Read the model definition and answer for the solid it produces. Units are mm, in the model's axes. A direction names the side the tool comes from. Coordinates: 2 decimals unless noted, no trailing zeros.
1) Each of these flat-tipped pins is pushed along its axis until it touches: pin 1 Ø15 at (x, y) = (-283.5, 99) entering from -Z; pin 2 Ø25 at (y, z) = (9.5, -34.5) entering from +X; pin 3 Ø15 at (y, z) = (-68.5, -71) entering from +X. Where does it stop, or does it pass through?
2) Find the intervals of material crossed by line 1 (Y direction, x = 168, z = -93); line 2 (Z direction, x = 123, y = 245), in increasing order.
3) The part is cut by section A-A (x = -170). Give the number of separate pieces and of enclosed holes in the cut face, then the cut area to 3 significant figures.
4) Determine the mould class of faces 1 (the face through (-300, -4, -25)), 2 (the face through (-4, 300, -25)), 3 (the face through (-5.91, 263.52, -677.54)), 4 (the face through (260.71, -239.53, -421.67)) for opening direction Y: +Y half, -Y half, draft (parallel to the pull), parting line (faces both ways), or undercut.
5) Which of the six approach directions +Z, -Z, +X, -X, +Y, -Y give full straight-line access (tool end or side, diameter ignored) to faces 5 (the face through (-254.688, -3, -75)), 6 (the face through (300, -4, -25)), 7 (the face through (3.72, -263.415, -676.431)), 8 (the face through (-295.762, 270.424, -751.192))?
from build123d import *

# Parameters (mm, degrees)
F0_W      = 50
F0_H      = 50
F2_W      = 50
F2_H      = 50
F3_W      = 600
F3_H      = 600
F8_DEPTH  = 50
F9_W      = 409.375
F9_H      = 409.375
F10_DEPTH = 50


with BuildPart() as f4:
    # F0 (on Top) → F4 section 0
    with BuildSketch(Plane.XY):
        with Locations((-225, -225)):
            Rectangle(F0_W, F0_H)
    # F2 (on offset) → F4 section 1
    with BuildSketch(Plane.XY.offset(-800)):
        with Locations((-300, -300)):
            Rectangle(F2_W, F2_H)
    loft()



with BuildPart() as f5:
    # F0 (on Top) → F5 section 0
    with BuildSketch(Plane.XY):
        with Locations((225, -225)):
            Rectangle(F0_W, F0_H)
    # F2 (on offset) → F5 section 1
    with BuildSketch(Plane.XY.offset(-800)):
        with Locations((300, -300)):
            Rectangle(F2_W, F2_H)
    loft()


with BuildPart() as f6:
    # F0 (on Top) → F6 section 0
    with BuildSketch(Plane.XY):
        with Locations((-225, 225)):
            Rectangle(F0_W, F0_H)
    # F2 (on offset) → F6 section 1
    with BuildSketch(Plane.XY.offset(-800)):
        with Locations((-300, 300)):
            Rectangle(F2_W, F2_H)
    loft()


with BuildPart() as f7:
    # F0 (on Top) → F7 section 0
    with BuildSketch(Plane.XY):
        with Locations((225, 225)):
            Rectangle(F0_W, F0_H)
    # F2 (on offset) → F7 section 1
    with BuildSketch(Plane.XY.offset(-800)):
        with Locations((300, 300)):
            Rectangle(F2_W, F2_H)
    loft()


with BuildPart() as f4_1:
    add(f4.part)

    add(f5.part)  # F8 merges F5

    add(f6.part)  # F8 merges F6

    add(f7.part)  # F8 merges F7
    # F3 (on Top) → F8 (join)
    with BuildSketch(Plane.XY):
        Rectangle(F3_W, F3_H)
    extrude(amount=-F8_DEPTH)

    # F9 (on face) → F10 (join)
    with BuildSketch(Plane(origin=(0, 0, -50), x_dir=(1, 0, 0), z_dir=(0, 0, -1))):
        Polygon((254.6875, -254.6875), (254.6875, -204.6875), (254.6875, 204.6875), (254.6875, 254.6875), (204.6875, 254.6875), (-204.6875, 254.6875), (-254.6875, 254.6875), (-254.6875, -254.6875), (-204.6875, -254.6875), (204.6875, -254.6875), align=None)
        Rectangle(F9_W, F9_H, mode=Mode.SUBTRACT)
    extrude(amount=F10_DEPTH)

    # F13 (on face) → F15 section 0
    with BuildSketch(Plane(origin=(-198.2575024201, 0, 18.5866408519), x_dir=(0, 1, 0), z_dir=(0.9956342261, 0, -0.0933407087))):
        Polygon((261.0594902568, -672.8252733026), (265.7063268379, -722.6088741144), (315.2744650336, -717.9821489666), (310.6276284526, -668.1985481548), align=None)
    # F14 (on face) → F15 section 1
    with BuildSketch(Plane(origin=(198.2575024201, 0, 18.5866408519), x_dir=(0, -1, 0), z_dir=(-0.9956342261, 0, -0.0933407087))):
        Polygon((-315.2744650336, -717.9821489666), (-265.7063268379, -722.6088741144), (-261.0594902568, -672.8252733026), (-310.6276284526, -668.1985481548), align=None)
    loft()

    # F12 (on face) → F18 section 0
    with BuildSketch(Plane(origin=(0, 198.2575024201, 18.5866408519), x_dir=(1, 0, 0), z_dir=(0, -0.9956342261, -0.0933407087))):
        Polygon((-315.7063268379, -722.6088741144), (-265.7063268379, -722.6088741144), (-261.0594902568, -672.8252733026), (-311.0594902568, -672.8252733026), align=None)
    # F16 (on face) → F18 section 1
    with BuildSketch(Plane(origin=(0, -198.2575024201, 18.5866408519), x_dir=(-1, 0, 0), z_dir=(0, 0.9956342261, -0.0933407087))):
        Polygon((261.0594902568, -672.8252733026), (265.7063268379, -722.6088741144), (315.7063268379, -722.6088741144), (311.0594902568, -672.8252733026), align=None)
    loft()

    # F17 (on face) → F21 section 0
    with BuildSketch(Plane(origin=(-198.2575024201, 0, 18.5866408519), x_dir=(0, 1, 0), z_dir=(0.9956342261, 0, -0.0933407087))):
        Polygon((-315.2744650336, -717.9821489666), (-265.7063268379, -722.6088741144), (-261.0594902568, -672.8252733026), (-310.6276284526, -668.1985481548), align=None)
    # F19 (on face) → F21 section 1
    with BuildSketch(Plane(origin=(198.2575024201, 0, 18.5866408519), x_dir=(0, -1, 0), z_dir=(-0.9956342261, 0, -0.0933407087))):
        Polygon((261.0594902568, -672.8252733026), (265.7063268379, -722.6088741144), (315.2744650336, -717.9821489666), (310.6276284526, -668.1985481548), align=None)
    loft()

    # F22 (on face) → F23 section 0
    with BuildSketch(Plane(origin=(0, 198.2575024201, 18.5866408519), x_dir=(1, 0, 0), z_dir=(0, -0.9956342261, -0.0933407087))):
        Polygon((261.0594902568, -672.8252733026), (265.7063268379, -722.6088741144), (315.7063268379, -722.6088741144), (311.0594902568, -672.8252733026), align=None)
    # F20 (on face) → F23 section 1
    with BuildSketch(Plane(origin=(0, -198.2575024201, 18.5866408519), x_dir=(-1, 0, 0), z_dir=(0, 0.9956342261, -0.0933407087))):
        Polygon((-315.2744650336, -717.9821489666), (-265.7063268379, -722.6088741144), (-261.0594902568, -672.8252733026), (-310.6276284526, -668.1985481548), align=None)
    loft()


solid = f4_1.part
Reported:
1. pin 1: stops at z = -700.87
1. pin 2: stops at x = 300
1. pin 3: stops at x = 254.69
2. line 1: y = -254.69 to -204.69, 204.69 to 254.69
2. line 2: z = -100 to 0
3. separate pieces: 3
3. enclosed holes: 0
3. area: 40,000 mm2
4. face 1: draft
4. face 2: +Y half
4. face 3: undercut
4. face 4: undercut
5. face 5: -Z, -X
5. face 6: +Z, +X, +Y, -Y
5. face 7: -Z
5. face 8: -Z, +X, -X
